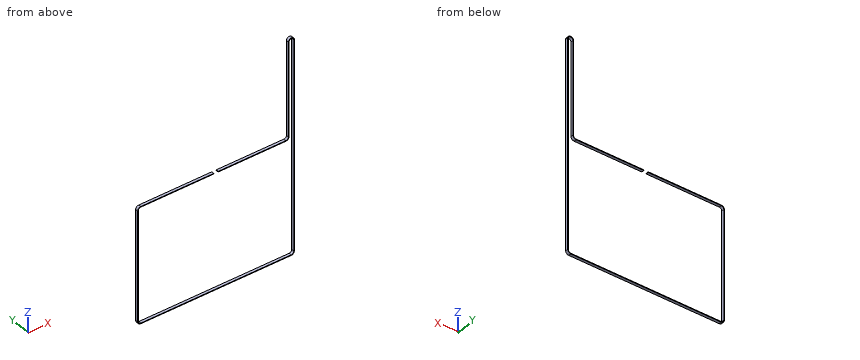
from build123d import *

# Parameters (mm, degrees)
EXTRUDE_THIN1_DEPTH = 6


with BuildPart() as part:
    # Sketch1 → Extrude-Thin1 (new body)
    with BuildSketch(Plane(origin=(0, 0, 0), x_dir=(1, 0, 0), z_dir=(0, 1, 0))):
        with BuildLine():
            Line((173.28, -259.643481844), (6.875, -259.643481844))
            ThreePointArc((6.875, -259.643481844), (2.723576088, -257.923905757), (1.004, -253.772481844))
            Line((1.004, -253.772481844), (1.004, -6.875))
            ThreePointArc((1.004, -6.875), (2.723576088, -2.723576088), (6.875, -1.004))
            Line((6.875, -1.004), (349.875, -1.004))
            ThreePointArc((349.875, -1.004), (354.026423912, -2.723576088), (355.746, -6.875))
            Line((355.746, -6.875), (355.746, -478.035))
            ThreePointArc((355.746, -478.035), (350.38, -483.401), (345.014, -478.035))
            Line((345.014, -478.035), (345.014, -267.017481844))
            ThreePointArc((345.014, -267.017481844), (342.854205404, -261.80327644), (337.64, -259.643481844))
            Line((337.64, -259.643481844), (183.275, -259.643481844))
            Line((183.275, -259.643481844), (183.275, -261.023481844))
            Line((183.275, -261.023481844), (337.64, -261.023481844))
            ThreePointArc((337.64, -261.023481844), (341.878398046, -262.779083798), (343.634, -267.017481844))
            Line((343.634, -267.017481844), (343.634, -478.035))
            ThreePointArc((343.634, -478.035), (350.38, -484.781), (357.126, -478.035))
            Line((357.126, -478.035), (357.126, -6.875))
            ThreePointArc((357.126, -6.875), (355.00223127, -1.74776873), (349.875, 0.376))
            Line((349.875, 0.376), (6.875, 0.376))
            ThreePointArc((6.875, 0.376), (1.74776873, -1.74776873), (-0.376, -6.875))
            Line((-0.376, -6.875), (-0.376, -253.772481844))
            ThreePointArc((-0.376, -253.772481844), (1.74776873, -258.899713115), (6.875, -261.023481844))
            Line((6.875, -261.023481844), (173.28, -261.023481844))
            Line((173.28, -261.023481844), (173.28, -259.643481844))
        make_face()
    extrude(amount=EXTRUDE_THIN1_DEPTH)


solid = part.part
Read the model definition and answer for the solid it produces. Units are mm, in the model's axes. Round coordinates to 2 decimals unless told otherwise and drop trailing zeros. Write each loop counter-clockwise with the first axis right and the second up, starting at its lowest first coordinate (ties: lowest second). Pieces come first, ordered by that corner, then holes.
1. Straight lines are drawn through the part: L1, parallel to Z at x = 251, y = 0.5; L2, parallel to X at y = 1.8, z = 226; L3, parallel to X at y = 1.05, z = 465. For each, find the intervals that lie inside material, in ascending order.
2. The part is cut by section C-C, the plane y = 5.05. Determine the outline of the cut face in (x, z) (3 decimals), then the cut area to 3 significant figures.
3. Given pin 1 Ø1.8 at (y, z) = (4.5, 340.5) entering from -X; pin 2 Ø0.7 at (y, z) = (4.5, 260) entering from -X, each flat-ended and moving along its own axis, determine where each tip first touches the part or whether it passes through.
4. The part is cut by section A-A, the plane x = 230. Determine the outline of the cut face in (y, z), then the cut area to 3 significant figures.
5. The part is cut by section B-B, the plane z = 354. Determine the outline of the cut face in (x, y), then the cut area to 3 significant figures.
Values:
1. L1: z = -0.38 to 1, 259.64 to 261.02
1. L2: x = -0.38 to 1, 355.75 to 357.13
1. L3: x = 343.63 to 345.01, 355.75 to 357.13
2. outline: (-0.376, 6.875) arc R7.251 ccw to (6.875, -0.376) - (349.875, -0.376) arc R7.251 ccw to (357.126, 6.875) - (357.126, 478.035) arc R6.746 ccw to (343.634, 478.035) - (343.634, 267.017) arc R5.994 cw to (337.64, 261.023) - (183.275, 261.023) - (183.275, 259.643) - (337.64, 259.643) arc R7.374 ccw to (345.014, 267.017) - (345.014, 478.035) arc R5.366 cw to (355.746, 478.035) - (355.746, 6.875) arc R5.871 cw to (349.875, 1.004) - (6.875, 1.004) arc R5.871 cw to (1.004, 6.875) - (1.004, 253.772) arc R5.871 cw to (6.875, 259.643) - (173.28, 259.643) - (173.28, 261.023) - (6.875, 261.023) arc R7.251 ccw to (-0.376, 253.772) - close
2. area: 2,280 mm2
3. pin 1: stops at x = 343.63
3. pin 2: stops at x = 2.63
4. outline: (0, -0.38) - (6, -0.38) - (6, 1) - (0, 1) - close; (0, 259.64) - (6, 259.64) - (6, 261.02) - (0, 261.02) - close
4. area: 16.6 mm2
5. outline: (343.63, 0) - (345.01, 0) - (345.01, 6) - (343.63, 6) - close; (355.75, 0) - (357.13, 0) - (357.13, 6) - (355.75, 6) - close
5. area: 16.6 mm2
